```python
from build123d import *

# Parameters (mm, degrees)
SKETCH1_W            = 21.5
SKETCH1_H            = 10.5
BOSS_EXTRUDE1_DEPTH  = 2
BOSS_EXTRUDE3_DEPTH  = 15
BOSS_EXTRUDE7_REACH  = 30.623
SKETCH8_W            = 1
SKETCH8_H            = 2
BOSS_EXTRUDE5_DEPTH  = 3
SKETCH6_R            = 1.7
BOSS_EXTRUDE6_DEPTH  = 2
BOSS_EXTRUDE8_DEPTH  = 2.5
FILLET1_R            = 1
SKETCH12_W           = 1
SKETCH12_H           = 10.5
CUT_EXTRUDE1_DEPTH   = 13
CUT_EXTRUDE2_DEPTH   = 1.5
SKETCH15_R           = 2.2
BOSS_EXTRUDE9_DEPTH  = 3
SKETCH16_R           = 0.670189152
BOSS_EXTRUDE10_DEPTH = 4.5
SKETCH17_R           = 2.2
CUT_EXTRUDE3_DEPTH   = 4.5
CUT_EXTRUDE4_START   = -4.5
SKETCH18_R           = 2.2
CUT_EXTRUDE4_DEPTH   = 4.5
FILLET2_R            = 6


with BuildPart() as part:
    # Sketch1 → Boss-Extrude1 (new body)
    with BuildSketch(Plane(origin=(0, 0, 0), x_dir=(1, 0, 0), z_dir=(0, 1, 0))):
        with Locations((10.75, 5.25)):
            Rectangle(SKETCH1_W, SKETCH1_H)
    extrude(amount=BOSS_EXTRUDE1_DEPTH)

    # Sketch3 → Boss-Extrude3 (add)
    with BuildSketch(Plane(origin=(0, 2, 0), x_dir=(1, 0, 0), z_dir=(0, 1, 0))):
        Polygon((0, 10.5), (22.5, 10.5), (22.5, 12), (-1, 12), (-1, -1.5), (22.5, -1.5), (22.5, 0), (0, 0), align=None)
    extrude(amount=-BOSS_EXTRUDE3_DEPTH)

    # Sketch8 → Boss-Extrude7 (add, up to next)
    with BuildSketch(Plane(origin=(0, 0, 0), x_dir=(-1, 0, 0), z_dir=(0, 0, -1)), mode=Mode.PRIVATE) as boss_extrude7_sk1:
        with Locations((-22, 1)):
            Rectangle(SKETCH8_W, SKETCH8_H)
    boss_extrude7_tool1 = extrude(boss_extrude7_sk1.sketch, amount=BOSS_EXTRUDE7_REACH, mode=Mode.PRIVATE) - part.part
    add(boss_extrude7_tool1.solids().sort_by_distance((22, 1, 0))[0])

    # Sketch5 → Boss-Extrude5 (add)
    with BuildSketch(Plane.XZ.offset(13)):
        Polygon((17.5, 0), (17.5, -10.5), (22.5, -10.5), (22.5, 1.5), (17.5, 1.5), align=None)
    extrude(amount=-BOSS_EXTRUDE5_DEPTH)



with BuildPart() as body_2:
    # Sketch6 → Boss-Extrude6 (new body)
    with BuildSketch(Plane.XY.offset(1.5)):
        with BuildLine():
            Line((22.5, 0), (22.5, 2))
            Line((22.5, 2), (17.24578851, 2))
            ThreePointArc((17.24578851, 2), (23.78286231, 11.271899542), (22.5, 0))
        make_face()
        with Locations((21.7, 5.8)):
            Circle(SKETCH6_R, mode=Mode.SUBTRACT)
    extrude(amount=-BOSS_EXTRUDE6_DEPTH)


with BuildPart() as part_1:
    add(part.part)

    add(body_2.part)  # Boss-Extrude8 merges body 2
    # Sketch9 → Boss-Extrude8 (add)
    with BuildSketch(Plane(origin=(0, 0, -0.5), x_dir=(-1, 0, 0), z_dir=(0, 0, -1))):
        with BuildLine():
            Line((-22.5, 2), (-22.577496439, 2))
            ThreePointArc((-22.577496439, 2), (-21.7, 9.7), (-20.822503561, 2))
            Line((-20.822503561, 2), (-17.24578851, 2))
            ThreePointArc((-17.24578851, 2), (-23.78286231, 11.271899542), (-22.5, 0))
            Line((-22.5, 0), (-22.5, 2))
        make_face()
    extrude(amount=BOSS_EXTRUDE8_DEPTH)

    # Fillet1
    fillet1_edges = [part_1.edges().sort_by_distance(p)[0] for p in [
        (22.5, 0, 0.75),
        (17.24578851, 2, -0.75),
    ]]
    fillet(fillet1_edges, radius=FILLET1_R)

    # Sketch12 → Cut-Extrude1 (cut)
    with BuildSketch(Plane.XZ.offset(13)):
        with Locations((-0.5, -5.25)):
            Rectangle(SKETCH12_W, SKETCH12_H)
    extrude(amount=-CUT_EXTRUDE1_DEPTH, mode=Mode.SUBTRACT)

    # Sketch13 → Cut-Extrude2 (cut)
    with BuildSketch(Plane.ZY.offset(1)):
        Polygon((-12, -13), (-12, 2), (1.5, 2), (1.5, -13), (0, -13), (0, 0), (-10.5, 0), (-10.5, -13), align=None)
    extrude(amount=-CUT_EXTRUDE2_DEPTH, mode=Mode.SUBTRACT)

    # Sketch15 → Boss-Extrude9 (add)
    with BuildSketch(Plane(origin=(0, 2, 0), x_dir=(1, 0, 0), z_dir=(0, 1, 0))):
        Polygon((5.85, 10.65), (16.65, 10.65), (16.65, -0.15), (16.65, -1.5), (2.6, -1.5), (2.6, 10.65), align=None)
        with Locations(Location((11.25, 5.25, 0), (0, 0, 270))):
            Circle(SKETCH15_R, mode=Mode.SUBTRACT)
    extrude(amount=BOSS_EXTRUDE9_DEPTH)

    # Sketch16 → Boss-Extrude10 (add)
    with BuildSketch(Plane.XY.offset(1.5)):
        with BuildLine():
            Line((2.6, 5), (2.6, 11.2))
            Line((2.6, 11.2), (19.4372583, 11.2))
            ThreePointArc((19.4372583, 11.2), (16.614535328, 8.701387439), (15.9, 5))
            Line((15.9, 5), (2.6, 5))
        make_face()
        with Locations((7.7, 5.8)):
            Circle(SKETCH16_R, mode=Mode.SUBTRACT)
    extrude(amount=-BOSS_EXTRUDE10_DEPTH)

    # Sketch17 → Cut-Extrude3 (cut)
    with BuildSketch(Plane.XY.offset(1.5)):
        with Locations((7.7, 5.8)):
            Circle(SKETCH17_R)
    extrude(amount=-CUT_EXTRUDE3_DEPTH, mode=Mode.SUBTRACT)

    # Sketch18 → Cut-Extrude4 (cut)
    with BuildSketch(Plane(origin=(0, 2, 0), x_dir=(1, 0, 0), z_dir=(0, 1, 0)).offset(CUT_EXTRUDE4_START)):
        with Locations(Location((11.25, 5.25, 0), (0, 0, 90))):
            Circle(SKETCH18_R)
    extrude(amount=CUT_EXTRUDE4_DEPTH, mode=Mode.SUBTRACT)

    # Fillet2
    fillet2_edges = [part_1.edges().sort_by_distance(p)[0] for p in [
        (2.6, 11.2, -0.75),
    ]]
    fillet(fillet2_edges, radius=FILLET2_R)


solid = part_1.part
```
Source: CAD feature listing. Evaluate the final solid. Frame: model axes, mm. A direction names the side the tool comes from. Give positions to 0.01 mm unless a question says otherwise; leave off trailing zeros. Order: outer loops, then holes, each group sorted by start corner. A loop starts at its lowest first (then second) coordinate and runs counter-clockwise, first axis right, second up. Notation, with made-up numbers: (84, 88.25) -> (102, 88.25) arc R13 ccw to (102, 105.25) -> close; hole circle Ø10 at (13, 87.5). An arc over 180 degrees is marked (long way). Use a Markdown table: item, result.
Q1. Section D-D (y = -2). Return the cut outline in (x, z).
A:
| item | result |
|---|---|
| outline | (0.5, -12) -> (22.5, -12) -> (22.5, -10.5) -> (0.5, -10.5) -> close; (0.5, 0) -> (22.5, 0) -> (22.5, 1.5) -> (0.5, 1.5) -> close |
Q2. Section B-B (z = -9). Return the cut outline in (x, y), and give its area (3 significant figures).
A:
| item | result |
|---|---|
| outline | (0.5, 0) -> (22.5, 0) -> (22.5, 2) -> (16.65, 2) -> (16.65, 5) -> (2.6, 5) -> (2.6, 2) -> (0.5, 2) -> close; (17.5, -13) -> (22.5, -13) -> (22.5, -10) -> (17.5, -10) -> close |
| area | 101 mm^2 |
Q3. Section A-A (x = 21.7). Return the cut outline in (y, z).
A:
| item | result |
|---|---|
| outline | (-13, -12) -> (2, -12) -> (2, -0.5) -> (4.1, -0.5) -> (4.1, 1.5) -> (-13, 1.5) -> close; (7.5, -0.5) -> (9.7, -0.5) -> (9.7, -3) -> (11.65, -3) -> (11.65, 1.5) -> (7.5, 1.5) -> close; hole (-10, -10.5) -> (0, -10.5) -> (0, 0) -> (-10, 0) -> close |
Q4. Material intervals for line 1 (Y direction, x = 21.7, z = -1.5); line 2 (X direction, y = 5.8, z = -1.55); line 3 (Z direction, x = 11.5, y = -6.5), sorted ascending. Write a range as [from, to].
A:
| item | result |
|---|---|
| line 1 | [-13, -10], [0, 2], [9.7, 11.65] |
| line 2 | [2.63, 5.5], [9.9, 17.8], [25.6, 27.55] |
| line 3 | [-12, -10.5], [0, 1.5] |
Q5. First-contact query: P1, Ø1.5, axis at x = 19.5, z = -6, coming from the +Y side; P2, Ø4, axis at x = 21.5, y = 6, coming from the -Z side; P3, Ø1.5, axis at y = 3, z = -5, coming from the +X side. Flat tips, straight axial feed; report the tip coordinate or a pass-through.
A:
| item | result |
|---|---|
| P1 | y = 2 |
| P2 | z = -0.5 |
| P3 | x = 16.65 |
Q6. Access query for faces 1 (the face through (16.65, 3, -7)), 2 (the face through (12, -7, 0)), 3 (the face through (10, 5, -8)), 4 (the face through (9.8, 6.46, -0.72)). Directions: +Z, -Z, +X, -X, +Y, -Y. A direction counts if a zero-diameter tool reaches every point of the face in a straight line with its end or side. Return the directions, or none.
A:
| item | result |
|---|---|
| face 1 | -Z, +X, +Y |
| face 2 | -X |
| face 3 | -Z, +X, -X, +Y |
| face 4 | +Z |
Q7. Pull-direction query (Y, two-part tool) for faces 5 (the face through (4.311, 9.396, -0.781)), 6 (the face through (12, -5, -12)), 7 (the face through (11, -7, -10.5)); classes: +Y half, -Y half, draft (parallel to the pull), parting line (faces both ways), or undercut.
A:
| item | result |
|---|---|
| face 5 | +Y half |
| face 6 | draft |
| face 7 | undercut |
Q8. Section C-C (x = 11.25). Return the cut outline in (y, z).
A:
| item | result |
|---|---|
| outline | (-13, -12) -> (2, -12) -> (2, -10.65) -> (5, -10.65) -> (5, -7.45) -> (0, -7.45) -> (0, -10.5) -> (-13, -10.5) -> close; (-13, 0) -> (0, 0) -> (0, -3.05) -> (5, -3.05) -> (5, -3) -> (11.2, -3) -> (11.2, 1.5) -> (-13, 1.5) -> close |
